The model under review builds one solid part; all positions refer to its coordinate system, in mm. Face numbers are marked on the shaded views. A direction names the side the tool comes from. Round coordinates to 2 decimals unless told otherwise and drop trailing zeros. Loops run counter-clockwise (first coordinate to the right, second up) from the corner with the lowest first, then second, coordinate; pieces in that order, holes last. Notation, with made-up numbers: (-33, -1.5) -> (2, -1.5) arc R10 cw to (2, 6.5) -> close; hole circle Ø5 at (3.25, 38). An arc over 180 degrees is marked (long way). Use a Markdown table: item, result. Add a question column.
1) For the marked faces 5, 6, 7 and 8, list the 3-axis set-ups (+Z, -Z, +X, -X, +Y, -Y) from which the entire face can be reached by the end or side of a thin tool; tool diameter is ignored.
2) Consider section B-B on z = 40.7. Give the boundary of the cut face in (x, y).
3) Consider section D-D on y = -88. Give the boundary of the cut face in (x, z).
4) Consider section C-C on y = -49.5. Give the boundary of the cut face in (x, z), plus the area to 3 significant figures.
5) Mouldability with a two-part tool opening along Z and no side actions: class the marked faces 1, 2, 3 and 4 as released by +Z, released by -Z, zero draft, split by the parting line, or undercut.
6) Insertion check: pin 1 (4.5 mm diameter, centred on y = 7, z = 40.5, fed in from +X); pin 2 (10 mm diameter, centred on x = 13.5, y = -73.5, fed in from +Z); pin 3 (10 mm diameter, centred on x = 23.5, y = -110.5, fed in from -Z); pin 4 (7 mm diameter, centred on y = 4.87, z = -11.3, fed in from -X). Each pin has a flat end and moves straight along its axis. Give the tip position at first contact, or say it passes through.
7) Wall thickness on probe 1 along Y at (x, z) = (18.5, -11.3); probe 2 along Z at (x, y) = (28.25, -41.5); probe 3 along Y at (x, z) = (25, -17): over which ranges is each line inside the solid? List them lowest first.
8) Consider section A-A on z = 14.7. Give the boundary of the cut face in (x, y), plus the area to 3 significant figures.
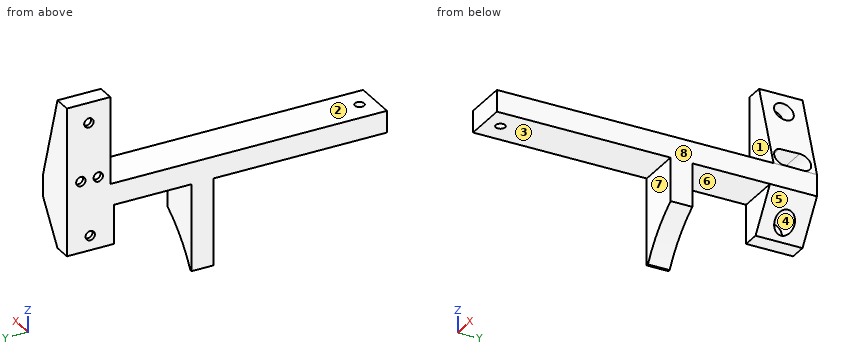
from build123d import *

# Parameters (mm, degrees)
SKETCH_1_W               = 20
SKETCH_1_H               = 147.415
SKETCH_1_R               = 2.15
EXTRUDE_1_DEPTH          = 10
SKETCH_2_W               = 20
SKETCH_2_H               = 20
EXTRUDE_2_DEPTH          = 40
SKETCH_3_W               = 20
SKETCH_3_H               = 21.635845778
EXTRUDE_3_DEPTH          = 18
CUT_EXTRUDE_1_DEPTH      = 10
CUT_EXTRUDE_1_DEPTH_BACK = 20
SKETCH_5_R               = 2.15
CUT_EXTRUDE_2_DEPTH      = 2
CUT_EXTRUDE_START        = -2
SKETCH_6_R               = 4.5
CUT_EXTRUDE_3_DEPTH      = 20
SKETCH_7_W               = 20
SKETCH_7_H               = 10
EXTRUDE_4_DEPTH          = 40
CUT_EXTRUDE_5_REACH      = 109.242


with BuildPart() as part:
    # 草图1 → 凸台-拉伸1 (new body)
    with BuildSketch(Plane.XY):
        with Locations((20.013762606, -58.095888527)):
            Rectangle(SKETCH_1_W, SKETCH_1_H)
        with Locations((20, -124.653388527)):
            Circle(SKETCH_1_R, mode=Mode.SUBTRACT)
    extrude(amount=EXTRUDE_1_DEPTH)

    # 草图2 → 凸台-拉伸2 (add)
    with BuildSketch(Plane.XY.offset(10)):
        with Locations((20.013762606, 5.611611473)):
            Rectangle(SKETCH_2_W, SKETCH_2_H)
    extrude(amount=EXTRUDE_2_DEPTH)

    # 草图3 → 凸台-拉伸3 (add)
    with BuildSketch(Plane(origin=(0, 0, 0), x_dir=(-1, 0, 0), z_dir=(0, 0, -1))):
        with Locations((-20.013762606, 4.793688584)):
            Rectangle(SKETCH_3_W, SKETCH_3_H)
    extrude(amount=EXTRUDE_3_DEPTH)

    # 草图4 → 切除-拉伸1 (cut, two sides: drawn at the far end of the back side and taken through both)
    with BuildSketch(Plane.XZ.offset(4.388388527).offset(-CUT_EXTRUDE_1_DEPTH_BACK)):
        Polygon((17.893762606, 50), (30.013762606, 50), (30.013762606, 10), align=None)
        Polygon((17.893762606, -18), (30.013762606, -18), (30.013762606, 0), align=None)
    extrude(amount=CUT_EXTRUDE_1_DEPTH + CUT_EXTRUDE_1_DEPTH_BACK, mode=Mode.SUBTRACT)

    # 草图5 → 切除-拉伸2 (cut)
    with BuildSketch(Plane.ZY.offset(-10.013762606)):
        with Locations(Location((14.7, 9.187302616, 0), (0, 0, 270))):
            Circle(SKETCH_5_R)
        with Locations(Location((14.7, 1.187302616, 0), (0, 0, 270))):
            Circle(SKETCH_5_R)
        with Locations(Location((40.7, 5.49974849, 0), (0, 0, 270))):
            Circle(SKETCH_5_R)
        with Locations(Location((-11.3, 4.874278045, 0), (0, 0, 270))):
            Circle(SKETCH_5_R)
    extrude(amount=-CUT_EXTRUDE_2_DEPTH, mode=Mode.SUBTRACT)

    # 草图6 → 切除-拉伸3 (cut)
    with BuildSketch(Plane.ZY.offset(-10.013762606).offset(CUT_EXTRUDE_START)):
        with Locations(Location((40.7, 5.49974849, 0), (0, 0, 270))):
            Circle(SKETCH_6_R)
        with Locations(Location((-11.3, 4.874278045, 0), (0, 0, 270))):
            Circle(SKETCH_6_R)
        with BuildLine():
            Line((19.2, 9.187302616), (18.942279399, -0.313718869))
            ThreePointArc((18.942279399, -0.313718869), (14.7, -3.312697384), (10.457720601, -0.313718869))
            Line((10.457720601, -0.313718869), (10.2, 9.187302616))
            ThreePointArc((10.2, 9.187302616), (14.7, 13.687302616), (19.2, 9.187302616))
        make_face()
    extrude(amount=-CUT_EXTRUDE_3_DEPTH, mode=Mode.SUBTRACT)

    # 草图7 → 凸台-拉伸4 (add)
    with BuildSketch(Plane(origin=(0, 0, 0), x_dir=(-1, 0, 0), z_dir=(0, 0, -1))):
        with Locations((-20.013762606, -46.803388527)):
            Rectangle(SKETCH_7_W, SKETCH_7_H)
    extrude(amount=EXTRUDE_4_DEPTH)

    # 草图8 → 切除-拉伸5 (cut, up to next)
    with BuildSketch(Plane(origin=(0, -41.803388527, 0), x_dir=(1, 0, 0), z_dir=(0, 1, 0)), mode=Mode.PRIVATE) as cut_extrude_5_sk1:
        with BuildLine():
            Line((30.013762606, 20), (30.013762606, 40))
            Line((30.013762606, 40), (11.013762606, 40))
            ThreePointArc((11.013762606, 40), (19.239482102, 28.789433521), (30.013762606, 20))
        make_face()
    cut_extrude_5_tool1 = extrude(cut_extrude_5_sk1.sketch, amount=-CUT_EXTRUDE_5_REACH, mode=Mode.PRIVATE) & part.part
    add(cut_extrude_5_tool1.solids().sort_by_distance((23.14433, -41.803389, -32.776655))[0], mode=Mode.SUBTRACT)


solid = part.part
Result set:
| question | item | result |
|---|---|---|
| 1 | face 5 | -Z, +X, +Y |
| 1 | face 6 | -Z, +X, -X |
| 1 | face 7 | -Z, +X, -X, -Y |
| 1 | face 8 | +Z, -Z, +X, +Y, -Y |
| 2 | outline | (10.01, -4.39) -> (20.71, -4.39) -> (20.71, 1) -> (12.01, 1) -> (12.01, 3.35) -> (10.01, 3.35) -> close; (10.01, 7.65) -> (12.01, 7.65) -> (12.01, 10) -> (20.71, 10) -> (20.71, 15.61) -> (10.01, 15.61) -> close |
| 3 | outline | (10.01, 0) -> (30.01, 0) -> (30.01, 10) -> (10.01, 10) -> close |
| 4 | outline | (10.01, -40) -> (11.01, -40) arc R55 cw to (30.01, -20) -> (30.01, 10) -> (10.01, 10) -> close |
| 4 | area | 778 mm2 |
| 5 | face 1 | zero draft |
| 5 | face 2 | released by +Z |
| 5 | face 3 | released by -Z |
| 5 | face 4 | undercut |
| 6 | pin 1 | x = 12.01 |
| 6 | pin 2 | z = 10 |
| 6 | pin 3 | z = 0 |
| 6 | pin 4 | x = 10.01 |
| 7 | probe 1 | -51.8 to -41.8, -6.02 to 0.37, 9.37 to 15.61 |
| 7 | probe 2 | 0 to 10 |
| 7 | probe 3 | -51.8 to -41.8 |
| 8 | outline | (10.01, -4.39) -> (28.59, -4.39) -> (28.59, -3.31) -> (12.01, -3.31) -> (12.01, -0.96) -> (10.01, -0.96) -> close; (10.01, 3.34) -> (12.01, 3.34) -> (12.01, 7.04) -> (10.01, 7.04) -> close; (10.01, 11.34) -> (12.01, 11.34) -> (12.01, 13.69) -> (28.59, 13.69) -> (28.59, 15.61) -> (10.01, 15.61) -> close |
| 8 | area | 72.5 mm2 |
